Design review of the part built by this model. Coordinates are the model's own, in mm. A direction names the side the tool comes from. Round coordinates to 2 decimals unless told otherwise and drop trailing zeros. Loops run counter-clockwise (first coordinate to the right, second up) from the corner with the lowest first, then second, coordinate; pieces in that order, holes last. Notation, with made-up numbers: (-34.5, 86) - (17.5, 86) arc R29 cw to (17.5, 108) - close; hole circle Ø7 at (65.25, 22). An arc over 180 degrees is marked (long way). Use one line per item in the form item = value. Start each with the question number.
(1) We need section B-B, the plane y = -34.14. Write out the cut boundary in (x, z).
(2) We need section D-D, the plane x = -27. Write out the cut boundary in (y, z), then the cut area to 3 significant figures.
(3) Machinability: for faces 1 (the flat face through (-1.5, 10, 1)), 2 (the flat face through (-34.5, -40, 6)), 3 (the flat face through (20.25, -40, 8)), 4 (the flat face through (-22, -44.34, 5)), which of the approach directions +Z, -Z, +X, -X, +Y, -Y give a long, thin tool a straight path to every point of the face, cutting with its end or side? Answer none if there is none.
(4) The part is to be moulded in two halves that separate along X. For faces 5 (the flat face through (-22, -68.34, 5)), 6 (the cylindrical face through (6.066, 17.515, 1.479)), 7 (the flat face through (1.5, 10, 1)), 8 (the flat face through (-29.25, -61, 5)), say which applies: released by +X, released by -X, zero draft, split by the parting line, or undercut.
(5) Wall thickness on probe 1 along Y at (x, z) = (-18.3, 1.1); probe 2 along Y at (x, z) = (-12.1, 2.2); probe 3 along X at (y, z) = (11, 2.5): over which ranges is each line inside the solid? List them lowest first. Write a range as [from, to].
(6) We need section C-C, the plane x = -18.3. Write out the cut boundary in (y, z).
(7) For pin 1 (2.5 mm diameter, centred on y = -12, z = 1, fed in from +X); pin 2 (4.5 mm diameter, centred on x = -12.1, y = -34.14, fed in from -Z); pin 3 (2 mm diameter, centred on y = -60, z = 6.5, fed in from -X); pin 4 (12 mm diameter, centred on x = -22, y = -56, fed in from +Z), all flat-tipped, find the tip position at first contact; note any pin that passes through.
(8) We need section A-A, the plane z = 11.5. Write out the cut boundary in (x, y).
from build123d import *

# Parameters (mm, degrees)
BOSS_EXTRUDE1_DEPTH = 3
SKETCH2_W           = 5.25
SKETCH2_H           = 30
BOSS_EXTRUDE2_DEPTH = 10
BOSS_EXTRUDE3_DEPTH = 4.5


with BuildPart() as part:
    # Sketch1 → Boss-Extrude1 (new body)
    with BuildSketch(Plane.XY):
        with BuildLine():
            Line((1.5, 0), (-1.5, 0))
            Line((-1.5, 0), (-1.5, 20))
            ThreePointArc((-1.5, 20), (-6.020163774, 17.572640687), (-7.5, 12.66))
            Line((-7.5, 12.66), (-7.5, 0))
            Line((-7.5, 0), (-7.5, -24.34))
            Line((-7.5, -24.34), (-34.5, -24.34))
            Line((-34.5, -24.34), (-34.5, -54.34))
            Line((-34.5, -54.34), (25.5, -54.34))
            Line((25.5, -54.34), (25.5, -24.34))
            Line((25.5, -24.34), (7.5, -24.34))
            Line((7.5, -24.34), (7.5, 0))
            Line((7.5, 0), (7.5, 12.66))
            ThreePointArc((7.5, 12.66), (6.020163774, 17.572640687), (1.5, 20))
            Line((1.5, 20), (1.5, 0))
        make_face()
        with BuildLine():
            ThreePointArc((-12.687903226, -31.50478278), (-24.5, -34.14), (-12.687903226, -36.77521722))
            ThreePointArc((-12.687903226, -36.77521722), (-9.4, -34.14), (-12.687903226, -31.50478278))
        make_face(mode=Mode.SUBTRACT)
    extrude(amount=BOSS_EXTRUDE1_DEPTH)

    # Sketch2 → Boss-Extrude2 (add)
    with BuildSketch(Plane.XY.offset(3)):
        with Locations((-31.875, -39.34)):
            Rectangle(SKETCH2_W, SKETCH2_H)
        with Locations((22.875, -39.34)):
            Rectangle(SKETCH2_W, SKETCH2_H)
    extrude(amount=BOSS_EXTRUDE2_DEPTH)

    # Sketch3 → Boss-Extrude3 (add)
    with BuildSketch(Plane.XY.offset(3)):
        Polygon((-29.25, -54.34), (-29.25, -44.34), (-14.25, -44.34), (-14.25, -68.34), (-29.25, -68.34), align=None)
    extrude(amount=BOSS_EXTRUDE3_DEPTH)


solid = part.part
Data:
q1.outline = (-34.5, 0) - (-24.5, 0) - (-24.5, 3) - (-29.25, 3) - (-29.25, 13) - (-34.5, 13) - close; (-9.4, 0) - (25.5, 0) - (25.5, 13) - (20.25, 13) - (20.25, 3) - (-9.4, 3) - close
q2.outline = (-68.34, 3) - (-54.34, 3) - (-54.34, 0) - (-24.34, 0) - (-24.34, 3) - (-44.34, 3) - (-44.34, 7.5) - (-68.34, 7.5) - close
q2.area = 198 mm^2
q3.face_1 = +Z, -Z, +Y
q3.face_2 = +Z, -Z, -X, +Y, -Y
q3.face_3 = +Z, +Y, -Y
q3.face_4 = +Z, +Y
q4.face_5 = zero draft
q4.face_6 = released by +X
q4.face_7 = undercut
q4.face_8 = released by -X
q5.probe_1 = [-54.34, -40.34], [-27.94, -24.34]
q5.probe_2 = [-54.34, -36.84], [-31.44, -24.34]
q5.probe_3 = [-7.5, -1.5], [1.5, 7.5]
q6.outline = (-68.34, 3) - (-54.34, 3) - (-54.34, 0) - (-40.34, 0) - (-40.34, 3) - (-44.34, 3) - (-44.34, 7.5) - (-68.34, 7.5) - close; (-27.94, 0) - (-24.34, 0) - (-24.34, 3) - (-27.94, 3) - close
q7.pin_1 = 7.5
q7.pin_2 = through
q7.pin_3 = -29.25
q7.pin_4 = 7.5
q8.outline = (-34.5, -54.34) - (-29.25, -54.34) - (-29.25, -24.34) - (-34.5, -24.34) - close; (20.25, -54.34) - (25.5, -54.34) - (25.5, -24.34) - (20.25, -24.34) - close
